The model under review builds one solid part; all positions refer to its coordinate system, in mm. A direction names the side the tool comes from. Give positions to 0.01 mm unless a question says otherwise; leave off trailing zeros. Order: outer loops, then holes, each group sorted by start corner. A loop starts at its lowest first (then second) coordinate and runs counter-clockwise, first axis right, second up. Notation, with made-up numbers: (0, 28.5) - (59, 28.5) arc R18 cw to (59, 35.5) - close; hole circle Ø2 at (5.25, 40.5). An arc over 180 degrees is marked (long way). Put each result on its own line as item: value.
```python
from build123d import *

# Parameters (mm, degrees)
BOSS_EXTRUDE1_DEPTH = 50
FILLET1_R           = 2
SKETCH2_R           = 6.5
SKETCH2_R_2         = 1.5
CUT_EXTRUDE1_DEPTH  = 20
SKETCH3_R           = 1.65
CUT_EXTRUDE2_DEPTH  = 20
FILLET2_R           = 1
FILLET3_R           = 1


with BuildPart() as part:
    # Sketch1 → Boss-Extrude1 (new body)
    with BuildSketch(Plane.XY):
        Polygon((0, 0), (0, 35), (5, 35), (5, 5), (40, 5), (40, 0), align=None)
    extrude(amount=BOSS_EXTRUDE1_DEPTH)

    # Fillet1
    fillet1_edges = [part.edges().sort_by_distance(p)[0] for p in [
        (0, 0, 25),
    ]]
    fillet(fillet1_edges, radius=FILLET1_R)

    # Sketch2 → Cut-Extrude1 (cut)
    with BuildSketch(Plane.ZY):
        with Locations((25, 12.7)):
            Circle(SKETCH2_R)
        with Locations((15.5, 12.7)):
            Circle(SKETCH2_R_2)
        with Locations((34.5, 12.7)):
            Circle(SKETCH2_R_2)
    extrude(amount=-CUT_EXTRUDE1_DEPTH, mode=Mode.SUBTRACT)

    # Sketch3 → Cut-Extrude2 (cut)
    with BuildSketch(Plane(origin=(0, 5, 0), x_dir=(1, 0, 0), z_dir=(0, 1, 0))):
        with Locations((20, -10)):
            Circle(SKETCH3_R)
        with Locations((20, -40)):
            Circle(SKETCH3_R)
    extrude(amount=-CUT_EXTRUDE2_DEPTH, mode=Mode.SUBTRACT)

    # Fillet2
    fillet2_edges = [part.edges().sort_by_distance(p)[0] for p in [
        (5, 5, 25),
    ]]
    fillet(fillet2_edges, radius=FILLET2_R)

    # Fillet3
    fillet3_edges = [part.edges().sort_by_distance(p)[0] for p in [
        (23, 5, 50),
        (0, 35, 25),
        (5, 35, 25),
        (40, 5, 25),
        (40, 0, 25),
        (2.5, 35, 50),
        (21, 0, 0),
        (21, 0, 50),
        (0, 18.5, 50),
        (0.585786438, 0.585786438, 0),
        (0.585786438, 0.585786438, 50),
        (5, 20.5, 0),
        (5, 20.5, 50),
        (5.292893219, 5.292893219, 0),
        (5.292893219, 5.292893219, 50),
        (0, 18.5, 0),
        (2.5, 35, 0),
        (40, 2.5, 50),
        (23, 5, 0),
        (40, 2.5, 0),
    ]]
    fillet(fillet3_edges, radius=FILLET3_R)


solid = part.part
```
(1) Wall thickness on L1, parallel to Z at x = 20, y = 3; L2, parallel to X at y = 3, z = 40; L3, parallel to Y at x = 2.9, z = 25: over which ranges is each line inside the solid? List them lowest first.
The answers:
L1: 0 to 8.35, 11.65 to 38.35, 41.65 to 50
L2: 0 to 18.35, 21.65 to 40
L3: 0 to 6.2, 19.2 to 35
(2) The part is to be moulded in two halves that separate along Z. For faces 1 (the flat face through (12, 3, 50)), 2 (the flat face through (12, 3, 0)), 3 (the flat face through (40, 3, 25)), 4 (the cylindrical face through (18.784, 2.535, 38.885)), say which applies: pulls with the +Z half, pulls with the -Z half, needs draft (parallel to the pull), parting line crosses it, or undercut.
The answers:
face 1: pulls with the +Z half
face 2: pulls with the -Z half
face 3: needs draft
face 4: undercut
(3) For faces 5 (the flat face through (2, 35, 25)), 6 (the flat face through (22, 5, 25)), list the 3-axis set-ups (+Z, -Z, +X, -X, +Y, -Y) from which the entire face can be reached by the end or side of a thin tool; tool diameter is ignored.
The answers:
face 5: +Z, -Z, +X, -X, +Y
face 6: +Z, -Z, +X, +Y
(4) Clearance check with flat-ended pins moving along their axes: pin 1 Ø15 at (y, z) = (12.7, 25) entering from +X; pin 2 Ø5 at (x, y) = (8.5, 13.5) entering from +Z; pin 3 Ø16.5 at (x, z) = (15, 15) entering from +Y; pin 4 Ø2 at (y, z) = (23, 43.5) entering from +X. State where each tip first meets the part, or that it passes through.
The answers:
pin 1: x = 5.4
pin 2: through
pin 3: y = 5
pin 4: x = 5
(5) Take a section at C-C, the plane x = 20. Write out the cut boundary in (y, z).
The answers:
outline: (0, 1) arc R1 ccw to (1, 0) - (4, 0) arc R1 ccw to (5, 1) - (5, 8.35) - (0, 8.35) - close; (0, 11.65) - (5, 11.65) - (5, 38.35) - (0, 38.35) - close; (0, 41.65) - (5, 41.65) - (5, 49) arc R1 ccw to (4, 50) - (1, 50) arc R1 ccw to (0, 49) - close
(6) Take a section at A-A, the plane z = 40. Write out the cut boundary in (x, y), then the cut area to 3 significant figures.
The answers:
outline: (0, 2) arc R2 ccw to (2, 0) - (18.35, 0) - (18.35, 5) - (6, 5) arc R1 cw to (5, 6) - (5, 34) arc R1 ccw to (4, 35) - (1, 35) arc R1 ccw to (0, 34) - close; (21.65, 0) - (39, 0) arc R1 ccw to (40, 1) - (40, 4) arc R1 ccw to (39, 5) - (21.65, 5) - close
area: 332 mm^2
(7) Take a section at B-B, the plane y = 18. Write out the cut boundary in (x, z), then the cut area to 3 significant figures.
The answers:
outline: (0, 1) arc R1 ccw to (1, 0) - (4, 0) arc R1 ccw to (5, 1) - (5, 21.24) - (0, 21.24) - close; (0, 28.76) - (5, 28.76) - (5, 49) arc R1 ccw to (4, 50) - (1, 50) arc R1 ccw to (0, 49) - close
area: 212 mm^2
(8) Take a section at D-D, the plane y = 31. Write out the cut boundary in (x, z).
The answers:
outline: (0, 1) arc R1 ccw to (1, 0) - (4, 0) arc R1 ccw to (5, 1) - (5, 49) arc R1 ccw to (4, 50) - (1, 50) arc R1 ccw to (0, 49) - close
